Check sheet for the modelled part. Datum: model origin and axes. Units: mm. Round coordinates to 2 decimals unless told otherwise and drop trailing zeros.
Item 1: Cross-section at A-A on z = 1.4. Count the separate pieces of the cut face and the enclosed holes in it, plus the area to 3 significant figures.
Item 2: Material ranges on line 1 (Y direction, x = 14, z = 3.5); line 2 (Y direction, x = -15, z = 4.35); line 3 (X direction, y = 15, z = 2.5), recorded low to high.
Item 3: Go/stop test with flat-tipped pins: pin 1 Ø2 at (x, z) = (13.5, 2) entering from -Y; pin 2 Ø1.5 at (x, z) = (-2, 2) entering from +Y (3 decimals); pin 3 Ø5 at (x, y) = (15.25, 15.25) entering from +Z. Record where each tip stops, or that it passes through.
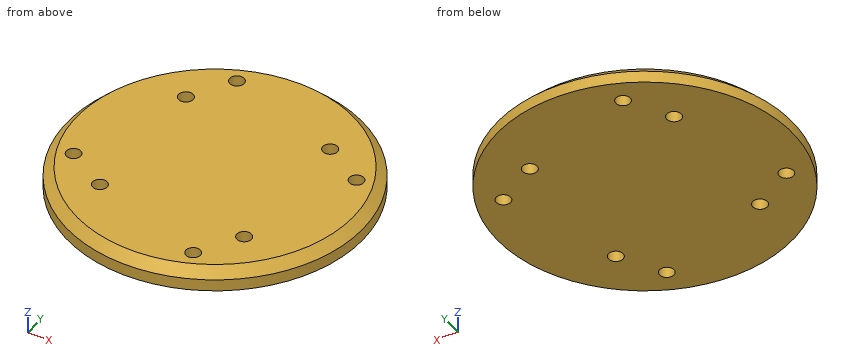
from build123d import *

# Parameters (mm, degrees)
F0_R            = 31.25
F1_DEPTH        = 4.5
F2_R            = 1.525
F3_DEPTH        = 4.501
F3_COPIES_COUNT = 4
F4_SIZE         = 2
F5_R            = 1.55
F6_DEPTH        = 4.501
F6_COPIES_COUNT = 4


# Not quite as in the source:
# - a pattern or mirror of a feature is missing from the dataset's text; its kind, count and spacing are read off the source's solid


with BuildPart() as f1:
    # F0 (on Top) → F1 (new body)
    with BuildSketch(Plane.XY):
        Circle(F0_R)
    extrude(amount=F1_DEPTH)

    # F2 (on face) → F3 (cut, through all)
    with BuildSketch(Plane.XY.offset(4.5)):
        with Locations((24.1067802187, 9.7397714288)):
            Circle(F2_R)
    f3 = extrude(amount=-F3_DEPTH, mode=Mode.SUBTRACT)

    # F3_copies: F3 ×4 about axis
    f3_copies_axis = Axis((0, 0, 0), (0, 0, 1))
    for i in range(1, F3_COPIES_COUNT):
        add(f3.rotate(f3_copies_axis, i * 360 / F3_COPIES_COUNT), mode=Mode.SUBTRACT)

    # F4
    f4_edges = [f1.edges().sort_by_distance(p)[0] for p in [
        (-31.25, 0, 4.5),
    ]]
    chamfer(f4_edges, length=F4_SIZE)

    # F5 (on face) → F6 (cut, through all)
    with BuildSketch(Plane.XY.offset(4.5)):
        with Locations((15.25, 15.25)):
            Circle(F5_R)
    f6 = extrude(amount=-F6_DEPTH, mode=Mode.SUBTRACT)

    # F6_copies: F6 ×4 about axis
    f6_copies_axis = Axis((0, 0, 0), (0, 0, 1))
    for i in range(1, F6_COPIES_COUNT):
        add(f6.rotate(f6_copies_axis, i * 360 / F6_COPIES_COUNT), mode=Mode.SUBTRACT)


solid = f1.part
Response values:
1. separate pieces: 1
1. enclosed holes: 8
1. area: 3,010 mm2
2. line 1: y = -26.82 to -16.17, -14.33 to 14.33, 16.17 to 26.82
2. line 2: y = -25.29 to -16.78, -13.72 to 13.72, 16.78 to 25.29
2. line 3: x = -27.41 to -16.78, -13.72 to 13.72, 16.78 to 27.41
3. pin 1: stops at y = -28.64
3. pin 2: stops at y = 31.225
3. pin 3: stops at z = 4.5
